Verification items for the finished model (mm, model axes). Face numbers are marked on the shaded views. A direction names the side the tool comes from. Round coordinates to 2 decimals unless told otherwise and drop trailing zeros. Order: outer loops, then holes, each group sorted by start corner. A loop starts at its lowest first (then second) coordinate and runs counter-clockwise, first axis right, second up. Notation, with made-up numbers: (10.25, 51) -> (31.25, 51) arc R19 cw to (31.25, 67) -> close; hole circle Ø4 at (6.25, 8.25). An arc over 180 degrees is marked (long way). Return JSON: item names as keys, results as strings. Group by question number.
1) Depth check by flat-ended pin: pin 1 (5 mm diameter, centred on y = -14, z = 2.5, fed in from +X); pin 2 (5 mm diameter, centred on x = 3, y = -3.5, fed in from -Z); pin 3 (2 mm diameter, centred on x = -1, y = -15, fed in from +Z). Enter the tip coordinate at first touch or a pass-through.
2) Scan lines: L1, parallel to Y at x = 2.25, z = 3; L2, parallel to Y at x = -1.75, z = 2.5; L3, parallel to X at y = -0.25, z = 0. Record each from-to range of solid material in increasing order.
3) Section check C-C on y = -11.5. Enter the section's corners in (x, z).
4) Section check D-D on z = -1.75. Enter the section's corners in (x, y).
5) Section check A-A on x = 0. Enter the section's corners in (y, z), plus the area to 3 significant figures.
6) Section check B-B on z = 0. Enter the section's corners in (x, y), plus the area to 4 significant figures.
7) Tool access check on the marked faces 1, 2 and 3. Record the directions out of +Z, -Z, +X, -X, +Y, -Y that give a thin tool (end or side, any length) a straight path to the whole face; none if there is none.
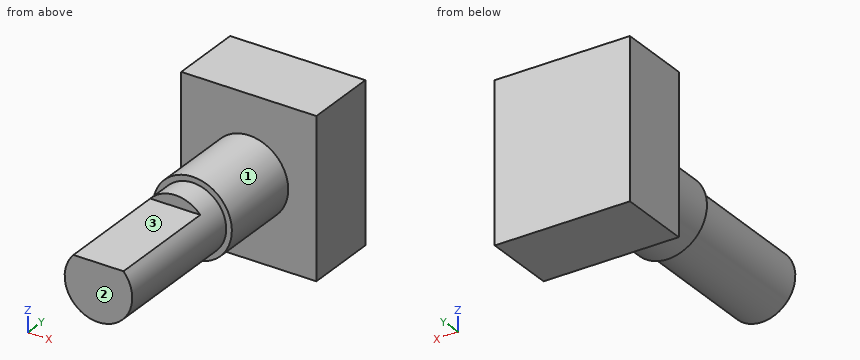
```python
from build123d import *

# Parameters (mm, degrees)
SKETCH1_W           = 12
SKETCH1_H           = 14
BOSS_EXTRUDE1_DEPTH = 6.5
SKETCH2_R           = 3.5
BOSS_EXTRUDE2_DEPTH = 7.5
SKETCH3_R           = 3
BOSS_EXTRUDE3_DEPTH = 12.5
CUT_EXTRUDE1_START  = -10.22
CUT_EXTRUDE1_DEPTH  = 10.22


with BuildPart() as part:
    # Sketch1 → Boss-Extrude1 (new body)
    with BuildSketch(Plane(origin=(0, 0, 0), x_dir=(1, 0, 0), z_dir=(0, 1, 0))):
        Rectangle(SKETCH1_W, SKETCH1_H)
    extrude(amount=BOSS_EXTRUDE1_DEPTH)

    # Sketch2 → Boss-Extrude2 (add)
    with BuildSketch(Plane.XZ):
        with Locations(Location((0, 0, 0), (0, 0, 90))):
            Circle(SKETCH2_R)
    extrude(amount=BOSS_EXTRUDE2_DEPTH)

    # Sketch3 → Boss-Extrude3 (add)
    with BuildSketch(Plane.XZ.offset(7.5)):
        with Locations(Location((0, 0, 0), (0, 0, 270))):
            Circle(SKETCH3_R)
    extrude(amount=BOSS_EXTRUDE3_DEPTH)

    # Sketch4 → Cut-Extrude1 (cut)
    with BuildSketch(Plane.XZ.offset(20).offset(CUT_EXTRUDE1_START)):
        with BuildLine():
            Line((-2.86, 2.017523234), (2.86, 2.017523234))
            ThreePointArc((2.86, 2.017523234), (0, 3.5), (-2.86, 2.017523234))
        make_face()
    extrude(amount=CUT_EXTRUDE1_DEPTH, mode=Mode.SUBTRACT)


solid = part.part
```
Check result:
{
 "1": {"pin 1": "x = 3", "pin 2": "z = -3.46", "pin 3": "z = 2.02"},
 "2": {"L1": "0 to 6.5", "L2": "-7.5 to 6.5", "L3": "-3.5 to 3.5"},
 "3": {"outline": "(-2.22, 2.02) arc R3 ccw (long way) to (2.22, 2.02) -> close"},
 "4": {"outline": "(-6, 0) -> (-3.03, 0) -> (-3.03, -7.5) -> (-2.44, -7.5) -> (-2.44, -20) -> (2.44, -20) -> (2.44, -7.5) -> (3.03, -7.5) -> (3.03, 0) -> (6, 0) -> (6, 6.5) -> (-6, 6.5) -> close"},
 "5": {"outline": "(-20, -3) -> (-7.5, -3) -> (-7.5, -3.5) -> (0, -3.5) -> (0, -7) -> (6.5, -7) -> (6.5, 7) -> (0, 7) -> (0, 3.5) -> (-7.5, 3.5) -> (-7.5, 3) -> (-9.78, 3) -> (-9.78, 2.02) -> (-20, 2.02) -> close", "area": "208 mm^2"},
 "6": {"outline": "(-6, 0) -> (-3.5, 0) -> (-3.5, -7.5) -> (-3, -7.5) -> (-3, -20) -> (3, -20) -> (3, -7.5) -> (3.5, -7.5) -> (3.5, 0) -> (6, 0) -> (6, 6.5) -> (-6, 6.5) -> close", "area": "205.5 mm^2"},
 "7": {"face 1": "-Y", "face 2": "+Z, -Z, +X, -X, -Y", "face 3": "+Z, +X, -X, -Y"}
}
